```python
from build123d import *

# Parameters (mm, degrees)
SKETCH1_W           = 11.34
SKETCH1_H           = 30
BOSS_EXTRUDE1_DEPTH = 3
CUT_EXTRUDE1_START  = -4
CUT_EXTRUDE1_DEPTH  = 5


with BuildPart() as part:
    # Sketch1 → Boss-Extrude1 (new body)
    with BuildSketch(Plane(origin=(0, 0, 0), x_dir=(1, 0, 0), z_dir=(0, 1, 0))):
        Rectangle(SKETCH1_W, SKETCH1_H)
    extrude(amount=BOSS_EXTRUDE1_DEPTH)

    # Sketch2 → Cut-Extrude1 (cut)
    with BuildSketch(Plane(origin=(0, 3, 0), x_dir=(1, 0, 0), z_dir=(0, 1, 0)).offset(CUT_EXTRUDE1_START)):
        Polygon((-5.145, -15), (-5.145, -0.77), (-5.67, 6.23), (-5.67, -15), align=None)
    cut_extrude1 = extrude(amount=CUT_EXTRUDE1_DEPTH, mode=Mode.SUBTRACT)

    # Mirror1: Cut-Extrude1 across plane
    add(cut_extrude1.mirror(Plane(origin=(0, 0, 0), x_dir=(0, 0, 1), z_dir=(1, 0, 0))), mode=Mode.SUBTRACT)


solid = part.part
```
Source: CAD feature listing. Evaluate the final solid. Frame: model axes, mm. A direction names the side the tool comes from. Give positions to 0.01 mm unless a question says otherwise; leave off trailing zeros. Write each loop counter-clockwise with the first axis right and the second up, starting at its lowest first coordinate (ties: lowest second). Pieces come first, ordered by that corner, then holes. Notation, with made-up numbers: (-13.5, -19) - (16.5, -19) arc R16 ccw to (16.5, 3) - close; hole circle Ø7 at (89, 36). An arc over 180 degrees is marked (long way). One line per item, written item: value. Start each with the question number.
Q1. Section query A-A, the plane y = 2.15. Return the cut outline in (x, z) (3 decimals), then the cut area to 3 significant figures.
Q2. Section query B-B, the plane z = 6.75. Return the cut outline in (x, y) (3 decimals).
Q3. Material intervals for probe 1 along X at (y, z) = (1.95, 7.25) (3 decimals); probe 2 along X at (y, z) = (2, -6), sorted ascending. Write a range as from..to.
Q4. Section query C-C, the plane z = 0. Return the cut outline in (x, y).
Q5. Set-up query: faces 1 (the face through (5.145, 1, 8)), 2 (the face through (-5.67, 1, -11)), 3 (the face through (-5.145, 1, 8)). Return all of +Z, -Z, +X, -X, +Y, -Y with unobstructed straight access to the full face (end or side cutting, diameter ignored); none if empty.
Answer:
1. outline: (-5.67, -15) - (5.67, -15) - (5.67, -6.23) - (5.145, 0.77) - (5.145, 15) - (-5.145, 15) - (-5.145, 0.77) - (-5.67, -6.23) - close
1. area: 322 mm2
2. outline: (-5.145, 0) - (5.145, 0) - (5.145, 3) - (-5.145, 3) - close
3. probe 1: x = -5.145..5.145
3. probe 2: x = -5.65..5.65
4. outline: (-5.2, 0) - (5.2, 0) - (5.2, 3) - (-5.2, 3) - close
5. face 1: +Z, +X, +Y, -Y
5. face 2: +Z, -Z, -X, +Y, -Y
5. face 3: +Z, -X, +Y, -Y
